Input: part model. Units: mm. Frame: model coordinates. A direction names the side the tool comes from. Give positions to 0.01 mm unless a question says otherwise; leave off trailing zeros. Order: outer loops, then holes, each group sorted by start corner. A loop starts at its lowest first (then second) coordinate and runs counter-clockwise, first axis right, second up. Notation, with made-up numbers: (86.25, 84.5) - (95.25, 84.5) arc R12 ccw to (95.25, 98.5) - close; hole circle Ø4 at (23.5, 47). An arc over 180 degrees is marked (long way). Use a Markdown table: item, result.
from build123d import *

# Parameters (mm, degrees)
SKETCH_1_W          = 20
SKETCH_1_H          = 20
EXTRUDE_1_DEPTH     = 90
SKETCH_2_W          = 20
SKETCH_2_H          = 90
EXTRUDE_2_DEPTH     = 20
SKETCH_4_W          = 34
SKETCH_4_H          = 90
CUT_EXTRUDE_1_DEPTH = 15
CUT_EXTRUDE_2_DEPTH = 15
SKETCH_8_R          = 5
CUT_EXTRUDE_3_DEPTH = 3
SKETCH_9_R          = 1.5
CUT_EXTRUDE_4_DEPTH = 5
CUT_EXTRUDE_5_DEPTH = 40
EXTRUDE_3_DEPTH     = 4
SKETCH_12_R         = 3
CUT_EXTRUDE_6_DEPTH = 2


with BuildPart() as part:
    # 草图1 → 凸台-拉伸1 (new body)
    with BuildSketch(Plane(origin=(0, 0, 0), x_dir=(1, 0, 0), z_dir=(0, 1, 0))):
        with Locations((10, -10)):
            Rectangle(SKETCH_1_W, SKETCH_1_H)
    extrude(amount=EXTRUDE_1_DEPTH)

    # 草图2 → 凸台-拉伸2 (add)
    with BuildSketch(Plane(origin=(0, 0, 0), x_dir=(-1, 0, 0), z_dir=(0, 0, -1))):
        with Locations((10, 45)):
            Rectangle(SKETCH_2_W, SKETCH_2_H)
    extrude(amount=-EXTRUDE_2_DEPTH)

    # 草图4 → 切除-拉伸1 (cut)
    with BuildSketch(Plane.XY.offset(20)):
        with Locations((-3, 45)):
            Rectangle(SKETCH_4_W, SKETCH_4_H)
    extrude(amount=-CUT_EXTRUDE_1_DEPTH, mode=Mode.SUBTRACT)

    # 草图6 → 切除-拉伸2 (cut)
    with BuildSketch(Plane(origin=(20, 0, 0), x_dir=(0, 0, -1), z_dir=(1, 0, 0))):
        with BuildLine():
            ThreePointArc((-10, 70.1), (-12.6, 67.5), (-10, 64.9))
            Line((-10, 64.9), (-10, 70.1))
        make_face()
        with BuildLine():
            Line((-10, 70.1), (-10, 64.9))
            ThreePointArc((-10, 64.9), (-8.161522369, 65.661522369), (-7.4, 67.5))
            ThreePointArc((-7.4, 67.5), (-8.161522369, 69.338477631), (-10, 70.1))
        make_face()
        with BuildLine():
            ThreePointArc((-7.4, 22.5), (-8.161522369, 24.338477631), (-10, 25.1))
            Line((-10, 25.1), (-10, 19.9))
            ThreePointArc((-10, 19.9), (-8.161522369, 20.661522369), (-7.4, 22.5))
        make_face()
        with BuildLine():
            Line((-10, 19.9), (-10, 25.1))
            ThreePointArc((-10, 25.1), (-12.6, 22.5), (-10, 19.9))
        make_face()
    extrude(amount=-CUT_EXTRUDE_2_DEPTH, mode=Mode.SUBTRACT)

    # 草图8 → 切除-拉伸3 (cut)
    with BuildSketch(Plane.ZY.offset(-14)):
        with Locations(Location((10, 67.5, 0), (0, 0, 270))):
            Circle(SKETCH_8_R)
        with Locations(Location((10, 22.5, 0), (0, 0, 270))):
            Circle(SKETCH_8_R)
    extrude(amount=-CUT_EXTRUDE_3_DEPTH, mode=Mode.SUBTRACT)

    # 草图9 → 切除-拉伸4 (cut)
    with BuildSketch(Plane.XY.offset(5)):
        with Locations((10, 65)):
            Circle(SKETCH_9_R)
        with Locations((10, 25)):
            Circle(SKETCH_9_R)
        with Locations((0, 65)):
            Circle(SKETCH_9_R)
        with Locations((0, 25)):
            Circle(SKETCH_9_R)
    extrude(amount=-CUT_EXTRUDE_4_DEPTH, mode=Mode.SUBTRACT)

    # 草图10 → 切除-拉伸5 (cut)
    with BuildSketch(Plane(origin=(0, 0, 0), x_dir=(-1, 0, 0), z_dir=(0, 0, -1))):
        with BuildLine():
            Line((0, 15), (-20, 15))
            Line((-20, 15), (-20, 0))
            Line((-20, 0), (20, 0))
            Line((20, 0), (20, 90))
            Line((20, 90), (-20, 90))
            Line((-20, 90), (-20, 75))
            Line((-20, 75), (0, 75))
            ThreePointArc((0, 75), (7.071067812, 72.071067812), (10, 65))
            Line((10, 65), (10, 25))
            ThreePointArc((10, 25), (7.071067812, 17.928932188), (0, 15))
        make_face()
    extrude(amount=-CUT_EXTRUDE_5_DEPTH, mode=Mode.SUBTRACT)

    # 草图11 → 凸台-拉伸3 (add)
    with BuildSketch(Plane(origin=(20, 0, 0), x_dir=(0, 0, -1), z_dir=(1, 0, 0))):
        Polygon((-6.95, 60), (-10, 60), (-13.05, 60), (-13.05, 30), (-10, 30), (-6.95, 30), align=None)
    extrude(amount=EXTRUDE_3_DEPTH)

    # 草图12 → 切除-拉伸6 (cut)
    with BuildSketch(Plane.XY.offset(5)):
        with Locations((0, 65)):
            Circle(SKETCH_12_R)
        with Locations((10, 65)):
            Circle(SKETCH_12_R)
        with Locations((0, 25)):
            Circle(SKETCH_12_R)
        with Locations((10, 25)):
            Circle(SKETCH_12_R)
    extrude(amount=-CUT_EXTRUDE_6_DEPTH, mode=Mode.SUBTRACT)


solid = part.part
1. Material intervals for line 1 along X through (y, z) = (65, 2.3); line 2 along Y through (x, z) = (10, 1.3); line 3 along Y through (x, z) = (15, 10), sorted ascending.
Response:
| item | result |
|---|---|
| line 1 | x = -10 to -1.5, 1.5 to 8.5, 11.5 to 20 |
| line 2 | y = 15 to 23.5, 26.5 to 63.5, 66.5 to 75 |
| line 3 | y = 15 to 17.5, 27.5 to 62.5, 72.5 to 75 |
2. Mould query, pull axis Y, two halves, no side actions, for faces 6 (the face through (17, 65, 8)), 7 (the face through (5, 45, 0)), 8 (the face through (22, 60, 10)). Classes: pulls with the +Y half, pulls with the -Y half, needs draft (parallel to the pull), parting line crosses it, or undercut.
Response:
| item | result |
|---|---|
| face 6 | undercut |
| face 7 | needs draft |
| face 8 | pulls with the +Y half |
3. Pin query (flat end, axial travel): pin 1 (1.2 mm diameter, centred on x = 22.5, y = 41, fed in from -Z); pin 2 (3 mm diameter, centred on x = -5.5, z = 2.5, fed in from -Y); pin 3 (5 mm diameter, centred on x = -4, y = 42.5, fed in from +Z); pin 4 (2.5 mm diameter, centred on x = 0, y = 65, fed in from -Z). Return the tip coordinate at first contact, or that it passes through.
Response:
| item | result |
|---|---|
| pin 1 | stops at z = 6.95 |
| pin 2 | stops at y = 15.83 |
| pin 3 | stops at z = 5 |
| pin 4 | passes through |
4. Set-up query: faces 1 (the face through (17, 20, 8)), 2 (the face through (1.3, 63.7, 3)), 3 (the face through (22, 45, 13.05)), 4 (the face through (22, 45, 6.95)), 5 (the face through (2, 45, 5)). Return all of +Z, -Z, +X, -X, +Y, -Y with unobstructed straight access to the full face (end or side cutting, diameter ignored); none if empty.
Response:
| item | result |
|---|---|
| face 1 | -X |
| face 2 | +Z |
| face 3 | +Z, +X, +Y, -Y |
| face 4 | -Z, +X, +Y, -Y |
| face 5 | +Z, -X, +Y, -Y |
5. Section query B-B (x = 10). Return loops of the section in (y, z), then the cut area to 3 significant figures.
Response:
| item | result |
|---|---|
| outline | (15, 0) - (23.5, 0) - (23.5, 3) - (22, 3) - (22, 5) - (15, 5) - close; (26.5, 0) - (63.5, 0) - (63.5, 3) - (62, 3) - (62, 5) - (28, 5) - (28, 3) - (26.5, 3) - close; (66.5, 0) - (75, 0) - (75, 5) - (68, 5) - (68, 3) - (66.5, 3) - close |
| area | 258 mm^2 |
6. Section query C-C (y = 50). Return loops of the section in (x, z), then the cut area to 3 significant figures.
Response:
| item | result |
|---|---|
| outline | (-10, 0) - (20, 0) - (20, 6.95) - (24, 6.95) - (24, 13.05) - (20, 13.05) - (20, 20) - (14, 20) - (14, 5) - (-10, 5) - close |
| area | 264 mm^2 |
7. Section query A-A (z = 4.25). Return loops of the section in (x, y).
Response:
| item | result |
|---|---|
| outline | (-10, 25) arc R10 ccw to (0, 15) - (20, 15) - (20, 75) - (0, 75) arc R10 ccw to (-10, 65) - close; hole circle Ø6 at (0, 25); hole circle Ø6 at (0, 65); hole circle Ø6 at (10, 25); hole circle Ø6 at (10, 65) |
8. Section query D-D (z = 9.25). Return loops of the section in (x, y), then the cut area to 3 significant figures.
Response:
| item | result |
|---|---|
| outline | (14, 15) - (20, 15) - (20, 20.01) - (17, 20.01) - (17, 17.56) - (14, 17.56) - close; (14, 27.44) - (17, 27.44) - (17, 24.99) - (20, 24.99) - (20, 30) - (24, 30) - (24, 60) - (20, 60) - (20, 65.01) - (17, 65.01) - (17, 62.56) - (14, 62.56) - close; (14, 72.44) - (17, 72.44) - (17, 69.99) - (20, 69.99) - (20, 75) - (14, 75) - close |
| area | 391 mm^2 |
